```python
from build123d import *

# Parameters (mm, degrees)
SKETCH1_W                    = 210
SKETCH1_H                    = 80
SKETCH1_R                    = 11.9875
SKETCH1_W_2                  = 26
SKETCH1_H_2                  = 51
BOSS_EXTRUDE1_DEPTH          = 6.35
M5_CLEARANCE_HOLE1_D         = 5.3
FILLET1_R                    = 5
TAP_DRILL_FOR_M8X1_25_TAP1_D = 6.8


with BuildPart() as part:
    # Sketch1 → Boss-Extrude1 (new body)
    with BuildSketch(Plane.XY):
        with Locations((35, 0)):
            Rectangle(SKETCH1_W, SKETCH1_H)
        Circle(SKETCH1_R, mode=Mode.SUBTRACT)
        with Locations((-50, 0)):
            Rectangle(SKETCH1_W_2, SKETCH1_H_2, mode=Mode.SUBTRACT)
        with Locations((120, 0)):
            Rectangle(SKETCH1_W_2, SKETCH1_H_2, mode=Mode.SUBTRACT)
    extrude(amount=-BOSS_EXTRUDE1_DEPTH)

    # M5 Clearance Hole1 (through all)
    with Locations(Plane(origin=(-30, 30, 0), x_dir=(1, 0, 0), z_dir=(0, 0, 1))):
        with Locations((0, 0), (0, -60), (130, -60), (130, 0)):
            Hole(M5_CLEARANCE_HOLE1_D / 2)

    # Fillet1
    fillet1_edges = [part.edges().sort_by_distance(p)[0] for p in [
        (-70, 40, -3.175),
        (140, 40, -3.175),
        (140, -40, -3.175),
        (-70, -40, -3.175),
    ]]
    fillet(fillet1_edges, radius=FILLET1_R)

    # Tap Drill for M8x1.25 Tap1 (through all)
    with Locations(Plane(origin=(-25, 12.5, 0), x_dir=(1, 0, 0), z_dir=(0, 0, 1))):
        with Locations((0, 0), (0, -25), (120, 0), (120, -25)):
            Hole(TAP_DRILL_FOR_M8X1_25_TAP1_D / 2)


solid = part.part
```
Geometry check sheet. Reference: the model listing, model coordinates, mm. A direction names the side the tool comes from. Give positions to 0.01 mm unless a question says otherwise; leave off trailing zeros. Loops run counter-clockwise (first coordinate to the right, second up) from the corner with the lowest first, then second, coordinate; pieces in that order, holes last. Notation, with made-up numbers: (33.25, 71.5) - (64.25, 71.5) arc R17 ccw to (64.25, 88.5) - close; hole circle Ø11 at (-33, 30.5). An arc over 180 degrees is marked (long way). Use CSV: the item, a comma, the result in double quotes. Start each with the question number.
Q1. Section check B-B, the plane y = 0. Record the cut outline in (x, z), and give its area (3 significant figures).
Q2. Scan lines: probe 1 along X at (y, z) = (-22, -1.75); probe 2 along Y at (x, z) = (95, -2.75); probe 3 along Y at (x, z) = (100, -2.75). Record each from-to range of solid material in increasing order. Write a range as from..to.
Q3. Section check C-C, the plane z = -2. Count the separate pieces of the cut face and the enclosed holes in it, and give its area (3 significant figures).
Q4. Section check A-A, the plane x = -25. Record the cut outline in (y, z), and give its area (3 significant figures).
Q5. Access from +Z, -Z, +X, -X, +Y, -Y to the whole of each face (thin tool, end or side, straight path). Record for faces 1 (the face through (-50, -25.5, -3)), 2 (the face through (140, 0, -3)).
Q6. Section check D-D, the plane y = 30. Record the cut outline in (x, z), and give its area (3 significant figures).
Q7. Release check for a two-part mould opening along X. For faces 3 (the face through (34, -40, -3)), 4 (the face through (138, 39, -3)), 5 (the face through (-70, 0, -3)), 6 (the face through (-28.047, 31.791, -3.219)) record: +X half, -X half, draft (parallel to the pull), parting line (faces both ways), or undercut.
Findings below:
1,outline,"(-70, -6.35) - (-63, -6.35) - (-63, 0) - (-70, 0) - close; (-37, -6.35) - (-11.99, -6.35) - (-11.99, 0) - (-37, 0) - close; (11.99, -6.35) - (107, -6.35) - (107, 0) - (11.99, 0) - close; (133, -6.35) - (140, -6.35) - (140, 0) - (133, 0) - close"
1,area,"851 mm^2"
2,probe 1,"x = -70..-63, -37..107, 133..140"
2,probe 2,"y = -40..-15.9, -9.1..9.1, 15.9..40"
2,probe 3,"y = -40..-32.65, -27.35..27.35, 32.65..40"
3,separate pieces,"1"
3,enclosed holes,"11"
3,area,"13,400 mm^2"
4,outline,"(-40, -6.35) - (-15.9, -6.35) - (-15.9, 0) - (-40, 0) - close; (-9.1, -6.35) - (9.1, -6.35) - (9.1, 0) - (-9.1, 0) - close; (15.9, -6.35) - (40, -6.35) - (40, 0) - (15.9, 0) - close"
4,area,"422 mm^2"
5,face 1,"+Z, -Z"
5,face 2,"+Z, -Z, +X, +Y, -Y"
6,outline,"(-70, -6.35) - (-32.65, -6.35) - (-32.65, 0) - (-70, 0) - close; (-27.35, -6.35) - (97.35, -6.35) - (97.35, 0) - (-27.35, 0) - close; (102.65, -6.35) - (140, -6.35) - (140, 0) - (102.65, 0) - close"
6,area,"1,270 mm^2"
7,face 3,"draft"
7,face 4,"+X half"
7,face 5,"-X half"
7,face 6,"undercut"
